Model file for the job. Use its own axes, mm. Face numbers are marked on the shaded views. Give positions to 0.01 mm unless a question says otherwise; leave off trailing zeros. Write each loop counter-clockwise with the first axis right and the second up, starting at its lowest first coordinate (ties: lowest second). Pieces come first, ordered by that corner, then holes. Notation, with made-up numbers: (60, 11) - (67, 11) arc R6 cw to (67, 16) - close; hole circle Ø1 at (5.25, 68.25). An arc over 180 degrees is marked (long way). One line per item, written item: value. Start each with the question number.
(1) Cut at C-C, the plane x = 52. List the corners of the cut face in (y, z), and give its area (3 significant figures).
(2) Probe L1, parallel to Y at x = 82, z = 107.5; L2, parallel to X at y = 12, z = 103.5; L3, parallel to X at y = 14.2, z = 103.1. List the from-to ranges inside material, lowest first.
(3) Cut at D-D, the plane y = 38. List the corners of the cut face in (x, z).
(4) Cut at A-A, the plane x = 82. List the corners of the cut face in (y, z).
(5) Mould opens along Y. For the marked faces 1, 2 and 3 say: pulls with the +Y half, pulls with the -Y half, needs draft (parallel to the pull), parting line crosses it, or undercut.
(6) Cut at B-B, the plane y = 52. List the corners of the cut face in (x, z), and give its area (3 significant figures).
(7) Drop flat-ended pins along their axis: P1, Ø1.2, axis at y = 103.5, z = 107, coming from the +X side; P2, Ø1.1, axis at y = 3.5, z = 109, coming from the -X side; P3, Ø3, axis at x = 65.5, z = 108.5, coming from the -Y side. Give the stop position or say it passes through.
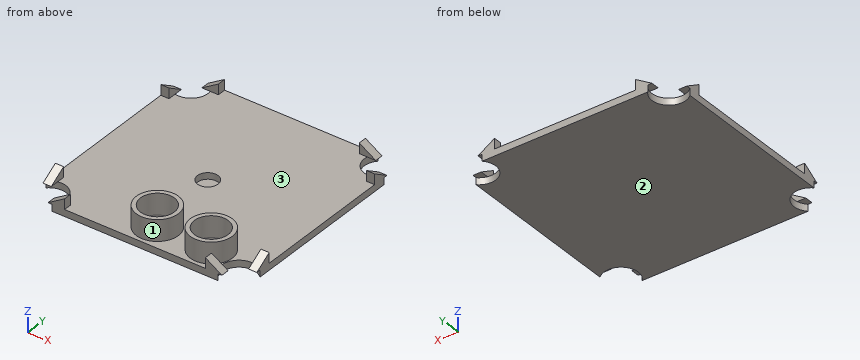
from build123d import *

# Parameters (mm, degrees)
SKETCH108_W     = 108
SKETCH108_H     = 108
PAD045_DEPTH    = 3.27
FILLET007_R     = 8
SKETCH_R        = 8.2
POCKET_DEPTH    = 3.271
SKETCH131_R     = 10.2
SKETCH131_R_2   = 8.2
PAD_DEPTH       = 10.2
SKETCH132_W     = 108
SKETCH132_H     = 108
POCKET052_DEPTH = 3.271
SKETCH133_R     = 5
POCKET053_DEPTH = 3.271
SKETCH134_W     = 4
SKETCH134_H     = 8
SKETCH134_W_2   = 8
SKETCH134_H_2   = 4
PAD052_DEPTH    = 5
POCKET054_DEPTH = 4
POCKET055_DEPTH = 4
POCKET056_DEPTH = 4
POCKET057_DEPTH = 4
SKETCH139_R     = 8.2
SKETCH139_R_2   = 5
PAD053_DEPTH    = 0.2


with BuildPart() as part:
    # Sketch108 → Pad045 (new body)
    with BuildSketch(Plane.XY):
        with Locations((54, 54)):
            Rectangle(SKETCH108_W, SKETCH108_H)
    extrude(amount=PAD045_DEPTH)

    # Fillet007
    fillet007_edges = [part.edges().sort_by_distance(p)[0] for p in [
        (0, 0, 1.635),
        (0, 108, 1.635),
        (108, 108, 1.635),
        (108, 0, 1.635),
    ]]
    fillet(fillet007_edges, radius=FILLET007_R)

    # Sketch (on Face5 of Fillet007) → Pocket (cut, through all)
    with BuildSketch(Plane.XY.offset(3.27)):
        with Locations((55.9, 14.2)):
            Circle(SKETCH_R)
        with Locations((82, 14.2)):
            Circle(SKETCH_R)
    extrude(amount=-POCKET_DEPTH, mode=Mode.SUBTRACT)

    # Sketch131 (on Face5 of Pocket) → Pad (join)
    with BuildSketch(Plane.XY.offset(3.27)):
        with Locations((55.9, 14.2)):
            Circle(SKETCH131_R)
        with Locations((55.9, 14.2)):
            Circle(SKETCH131_R_2, mode=Mode.SUBTRACT)
        with Locations((82, 14.2)):
            Circle(SKETCH131_R)
        with Locations((82, 14.2)):
            Circle(SKETCH131_R_2, mode=Mode.SUBTRACT)
    extrude(amount=PAD_DEPTH)

    # Sketch132 (on Face5 of Pad) → Pocket052 (cut, through all)
    with BuildSketch(Plane.XY.offset(3.27)):
        with Locations((54, 54)):
            Rectangle(SKETCH132_W, SKETCH132_H)
        with BuildLine():
            Line((2.25, 94.088366), (2.25, 13.918289))
            ThreePointArc((13.91388, 2.25), (13.833782, 13.833813), (2.25, 13.918289))
            Line((13.91388, 2.25), (94.083957, 2.25))
            ThreePointArc((105.75, 13.916052), (94.167504, 13.832496), (94.083957, 2.25))
            Line((105.75, 94.086129), (105.75, 13.916052))
            ThreePointArc((94.085398, 105.75), (94.217085, 94.217093), (105.75, 94.086129))
            Line((13.915321, 105.75), (94.085398, 105.75))
            ThreePointArc((2.25, 94.088366), (13.766826, 94.233221), (13.915321, 105.75))
        make_face(mode=Mode.SUBTRACT)
    extrude(amount=-POCKET052_DEPTH, mode=Mode.SUBTRACT)

    # Sketch133 (on Face1 of Pocket052) → Pocket053 (cut, through all)
    with BuildSketch(Plane.XY.offset(3.27)):
        with Locations((52, 52)):
            Circle(SKETCH133_R)
    extrude(amount=-POCKET053_DEPTH, mode=Mode.SUBTRACT)

    # Sketch134 (on Face1 of Pocket053) → Pad052 (join)
    with BuildSketch(Plane.XY.offset(3.27)):
        with Locations((4.25, 92.088366)):
            Rectangle(SKETCH134_W, SKETCH134_H)
        with Locations((15.915321, 103.75)):
            Rectangle(SKETCH134_W_2, SKETCH134_H_2)
        with Locations((92.085398, 103.75)):
            Rectangle(SKETCH134_W_2, SKETCH134_H_2)
        with Locations((103.75, 92.086129)):
            Rectangle(SKETCH134_W, SKETCH134_H)
        with Locations((103.75, 15.916052)):
            Rectangle(SKETCH134_W, SKETCH134_H)
        with Locations((92.083957, 4.25)):
            Rectangle(SKETCH134_W_2, SKETCH134_H_2)
        with Locations((15.91388, 4.25)):
            Rectangle(SKETCH134_W_2, SKETCH134_H_2)
        with Locations((4.25, 15.918289)):
            Rectangle(SKETCH134_W, SKETCH134_H)
    extrude(amount=PAD052_DEPTH)

    # Sketch135 (on Face24 of Pad052) → Pocket054 (cut)
    with BuildSketch(Plane.YZ.offset(105.75)):
        Polygon((96.086129, 8.27), (88.086129, 8.27), (96.086129, 3.27), align=None)
        Polygon((11.916052, 8.27), (19.916052, 8.27), (11.916052, 3.27), align=None)
    extrude(amount=-POCKET054_DEPTH, mode=Mode.SUBTRACT)

    # Sketch136 (on Face27 of Pocket054) → Pocket055 (cut)
    with BuildSketch(Plane(origin=(0, 105.75, 0), x_dir=(-1, 0, 0), z_dir=(0, 1, 0))):
        Polygon((-96.085398, 8.27), (-88.085398, 8.27), (-96.085398, 3.27), align=None)
        Polygon((-19.915321, 8.27), (-11.915321, 8.27), (-11.915321, 3.27), align=None)
    extrude(amount=-POCKET055_DEPTH, mode=Mode.SUBTRACT)

    # Sketch137 (on Face18 of Pocket055) → Pocket056 (cut)
    with BuildSketch(Plane(origin=(2.25, 0, 0), x_dir=(0, -1, 0), z_dir=(-1, 0, 0))):
        Polygon((-96.088366, 8.27), (-88.088366, 8.27), (-96.088366, 3.27), align=None)
        Polygon((-19.918289, 8.27), (-11.918289, 8.27), (-11.918289, 3.27), align=None)
    extrude(amount=-POCKET056_DEPTH, mode=Mode.SUBTRACT)

    # Sketch138 (on Face17 of Pocket056) → Pocket057 (cut)
    with BuildSketch(Plane.XZ.offset(-2.25)):
        Polygon((11.91388, 8.27), (19.91388, 8.27), (11.91388, 3.27), align=None)
        Polygon((88.083957, 8.27), (96.083957, 8.27), (96.083957, 3.27), align=None)
    extrude(amount=-POCKET057_DEPTH, mode=Mode.SUBTRACT)

    # Sketch139 (on Face1 of Pocket057) → Pad053 (join)
    with BuildSketch(Plane(origin=(0, 0, 0), x_dir=(1, 0, 0), z_dir=(0, 0, -1))):
        with Locations((55.9, -14.2)):
            Circle(SKETCH139_R)
        with Locations((82, -14.2)):
            Circle(SKETCH139_R)
        with Locations((52, -52)):
            Circle(SKETCH139_R_2)
    extrude(amount=-PAD053_DEPTH)


with BuildPart() as part_1:
    # Body020 placement: moved
    add(part.part.moved(Location((0, 0, 102))))


solid = part_1.part
Answers follow:
1. outline: (2.25, 102) - (105.75, 102) - (105.75, 105.27) - (57, 105.27) - (57, 102.2) - (47, 102.2) - (47, 105.27) - (23.62, 105.27) - (23.62, 115.47) - (21.41, 115.47) - (21.41, 102.2) - (6.99, 102.2) - (6.99, 115.47) - (4.78, 115.47) - (4.78, 105.27) - (2.25, 105.27) - close
1. area: 309 mm²
2. L1: y = 4 to 6, 22.4 to 24.4
2. L2: x = 15.22 to 48, 63.8 to 74.1, 89.9 to 92.79
2. L3: x = 2.25 to 2.55, 13.44 to 47.7, 64.1 to 73.8, 90.2 to 94.56, 105.44 to 105.75
3. outline: (2.25, 102) - (105.75, 102) - (105.75, 105.27) - (2.25, 105.27) - close
4. outline: (2.25, 102) - (105.75, 102) - (105.75, 105.27) - (24.4, 105.27) - (24.4, 115.47) - (22.4, 115.47) - (22.4, 102.2) - (6, 102.2) - (6, 115.47) - (4, 115.47) - (4, 105.27) - (2.25, 105.27) - close
5. face 1: parting line crosses it
5. face 2: needs draft
5. face 3: undercut
6. outline: (2.25, 102) - (105.75, 102) - (105.75, 105.27) - (57, 105.27) - (57, 102.2) - (47, 102.2) - (47, 105.27) - (2.25, 105.27) - close
6. area: 308 mm²
7. P1: stops at x = 94.28
7. P2: stops at x = 17
7. P3: stops at y = 8
